Answer from the drawing. Dimensions are ordinates in mm from the lowest x, y and z of the part. A direction names the side the tool comes from. Coordinates: 2 decimals unless noted, no trailing zeros. Order: outer loops, then holes, each group sorted by start corner. A loop starts at its lowest first (then second) coordinate and runs counter-clockwise, first axis right, second up. Notation, with made-up numbers: (55.5, 70) - (66.5, 70) arc R22 cw to (66.5, 91) - close; hole circle Ø10 at (13, -20.5). An arc over 180 degrees is marked (long way). Answer as a JSON object with one key per item and string values. Group by question number.
1) The mould has two halves that part along X. Classify the marked faces 3, 4 and 5: released by +X, released by -X, zero draft, split by the parting line, or undercut.
2) Section A-A (y = 2.25) is taken. Give the vertices of the cut face in (x, z).
3) Section D-D (y = 3.25) is taken. Give the vertices of the cut face in (x, z).
4) A tool of negligible diameter and unlimited length cuts with its end or side. For the marked faces 1 and 2, from which of +Z, -Z, +X, -X, +Y, -Y can it reach the whole face along a straight path? Write none if from no direction.
5) Section C-C (x = 5) is taken. Give the vertices of the cut face in (y, z).
6) Section B-B (z = 5) is taken. Give the vertices of the cut face in (x, y).
7) Each of these flat-tipped pins is pushed along its axis until it touches: P1, Ø5, axis at x = 12, z = 4.5, coming from the +Y side; P2, Ø3.5, axis at y = 5, z = 5, coming from the -X side. Where does it stop, or does it pass through?
8) Find the intervals of material crossed by line 1 along X through (y, z) = (2.5, 0.5); line 2 along X through (y, z) = (0.4, 5); line 3 along Y through (x, z) = (17, 6), in increasing order.
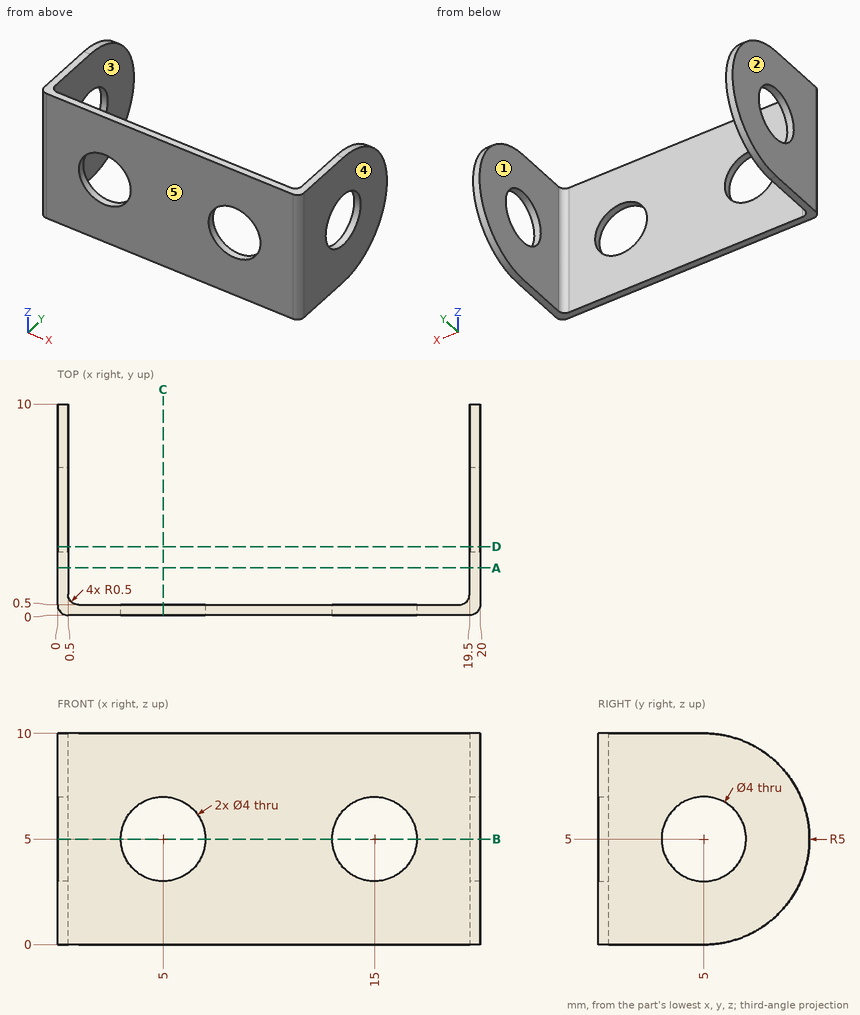
Report:
{
 "1": {"face 3": "undercut", "face 4": "released by +X", "face 5": "zero draft"},
 "2": {"outline": "(0, 0) - (0.5, 0) - (0.5, 10) - (0, 10) - close; (19.5, 0) - (20, 0) - (20, 10) - (19.5, 10) - close"},
 "3": {"outline": "(0, 0) - (0.5, 0) - (0.5, 4.03) - (0, 4.03) - close; (0, 5.97) - (0.5, 5.97) - (0.5, 10) - (0, 10) - close; (19.5, 0) - (20, 0) - (20, 4.03) - (19.5, 4.03) - close; (19.5, 5.97) - (20, 5.97) - (20, 10) - (19.5, 10) - close"},
 "4": {"face 1": "+Z, -Z, +Y", "face 2": "+Z, -Z, -X, +Y, -Y"},
 "5": {"outline": "(0, 0) - (0.5, 0) - (0.5, 3) - (0, 3) - close; (0, 7) - (0.5, 7) - (0.5, 10) - (0, 10) - close"},
 "6": {"outline": "(0, 0.5) arc R0.5 ccw to (0.5, 0) - (3, 0) - (3, 0.5) - (1, 0.5) arc R0.5 cw to (0.5, 1) - (0.5, 3) - (0, 3) - close; (0, 7) - (0.5, 7) - (0.5, 10) - (0, 10) - close; (7, 0) - (13, 0) - (13, 0.5) - (7, 0.5) - close; (17, 0) - (19.5, 0) arc R0.5 ccw to (20, 0.5) - (20, 3) - (19.5, 3) - (19.5, 1) arc R0.5 cw to (19, 0.5) - (17, 0.5) - close; (19.5, 7) - (20, 7) - (20, 10) - (19.5, 10) - close"},
 "7": {"P1": "stops at y = 0.5", "P2": "passes through"},
 "8": {"line 1": "x = 0 to 0.5, 19.5 to 20", "line 2": "x = 0.01 to 3, 7 to 13, 17 to 19.99", "line 3": "y = 0 to 0.5"}
}
